```python
from build123d import *

# Parameters (mm, degrees)
BOSS_EXTRUDE1_DEPTH             = 52
BOSS_EXTRUDE2_DEPTH             = 22
BOSS_EXTRUDE3_DEPTH             = 12
F_1_0MM_CLEARANCE_DOWEL_HOLE1_D = 18
FILLET1_R                       = 15


with BuildPart() as part:
    # Sketch1 → Boss-Extrude1 (new body)
    with BuildSketch(Plane.XY):
        with BuildLine():
            Line((0, -34), (-108, -34))
            ThreePointArc((-108, -34), (-142, 0), (-108, 34))
            Line((-108, 34), (0, 34))
            ThreePointArc((0, 34), (34, 0), (0, -34))
        make_face()
        with BuildLine():
            Line((0, -15), (-108, -15))
            ThreePointArc((-108, -15), (-123, 0), (-108, 15))
            Line((-108, 15), (0, 15))
            ThreePointArc((0, 15), (15, 0), (0, -15))
        make_face(mode=Mode.SUBTRACT)
    extrude(amount=BOSS_EXTRUDE1_DEPTH)

    # Sketch2 → Boss-Extrude2 (add)
    with BuildSketch(Plane.XY):
        with BuildLine():
            Line((-126.998451924, 28.196787485), (0, 28.196787485))
            Line((0, 28.196787485), (31.319910556, 13.231145179))
            Line((31.319910556, 13.231145179), (31.319910556, 76))
            ThreePointArc((31.319910556, 76), (14.710725641, 103.650160006), (-17.500876911, 101.974143))
            Line((-17.500876911, 101.974143), (-126.998451924, 28.196787485))
        make_face()
    extrude(amount=BOSS_EXTRUDE2_DEPTH)

    # Sketch3 → Boss-Extrude3 (add)
    with BuildSketch(Plane.XY.offset(22)):
        with BuildLine():
            Line((-31.319910556, 76), (-31.319910556, 27.253285183))
            Line((-31.319910556, 27.253285183), (31.319910556, 13.231145179))
            Line((31.319910556, 13.231145179), (31.319910556, 76))
            ThreePointArc((31.319910556, 76), (0, 107.319910556), (-31.319910556, 76))
        make_face()
    extrude(amount=BOSS_EXTRUDE3_DEPTH)

    # Ø1.0mm Clearance Dowel Hole1 (through all)
    with Locations(Plane.XY.offset(34)):
        with Locations((0, 76)):
            Hole(F_1_0MM_CLEARANCE_DOWEL_HOLE1_D / 2)

    # Fillet1
    fillet1_edges = [part.edges().sort_by_distance(p)[0] for p in [
        (-31.319910556, 34, 28),
    ]]
    fillet(fillet1_edges, radius=FILLET1_R)


solid = part.part
```
The listing builds one solid part. Answer for the finished solid, in the listing's coordinates (mm). A direction names the side the tool comes from. Give positions to 0.01 mm unless a question says otherwise; leave off trailing zeros. Loops run counter-clockwise (first coordinate to the right, second up) from the corner with the lowest first, then second, coordinate; pieces in that order, holes last. Notation, with made-up numbers: M 64.5,30 L 76.5,30 A18 cw 76.5,65 Z; hole C -24.5,24.5 d2. An arc over 180 degrees is marked long. One line per item, written item: value.
Q1. For faces 1 (the face through (-35.6, 38.51, 27.92)), 2 (the face through (31.32, 44, 17)), 3 (the face through (15, 0, 26)), 4 (the face through (32.2, -10.92, 25.64)), determine the directions among +Z, -Z, +X, -X, +Y, -Y from which every point of the face is accessible in a straight line to the end or side of a thin tool.
Working result:
face 1: +Z, -X, +Y
face 2: +Z, -Z, +X, +Y
face 3: +Z, -Z
face 4: +Z, +X
Q2. A cutting plane is placed at A-A on y = 0. Determine the outline of the cut face in (x, z).
Working result:
outline: M -142,0 L -123,0 L -123,52 L -142,52 Z; M 15,0 L 34,0 L 34,52 L 15,52 Z
Q3. Find the intervals of material crossed by line 1 (Y direction, x = -6, z = 29); line 2 (X direction, y = -11, z = 32); line 3 (Z direction, x = -12, y = 74.5), in increasing order. Write a range as from..to.
Working result:
line 1: y = -34..-15, 15..69.29, 82.71..106.74
line 2: x = -140.17..-118.2, 10.2..32.17
line 3: z = 0..34
Q4. A cutting plane is placed at D-D on y = 87. Determine the outline of the cut face in (x, z).
Working result:
outline: M -39.72,0 L 29.32,0 L 29.32,34 L -29.32,34 L -29.32,22 L -39.72,22 Z
Q5. A cutting plane is placed at C-C on x = -104. Determine the outline of the cut face in (y, z), then the cut area to 3 significant figures.
Working result:
outline: M -34,0 L -15,0 L -15,52 L -34,52 Z; M 15,0 L 43.69,0 L 43.69,22 L 34,22 L 34,52 L 15,52 Z
area: 2,190 mm^2
Q6. Determine the mould class of faces 5 (the face through (-60, 54, 22)), 6 (the face through (1.951, 67.214, 16.762)), 7 (the face through (-141.99, -0.75, 25.64)) for opening direction Y: +Y half, -Y half, draft (parallel to the pull), parting line (faces both ways), or undercut.
Working result:
face 5: draft
face 6: undercut
face 7: parting line
Q7. Flat-ended cylindrical pins translate along their axes: P1, Ø3.5, axis at y = 69, z = 27.5, coming from the -X side; P2, Ø5, axis at x = -26.5, z = 44.5, coming from the +Y side; P3, Ø20.5, axis at x = 0, y = 76, coming from the +Z side. Find the tip coordinate at first contact, or state that the pin passes through.
Working result:
P1: stops at x = -31.32
P2: stops at y = 34
P3: stops at z = 34
Q8. A cutting plane is placed at B-B on z = 28. Determine the outline of the cut face in (x, y).
Working result:
outline: M -108,-34 L 0,-34 A34 ccw 31.32,13.23 L 31.32,76 A31.32 ccw -31.32,76 L -31.32,49 A15 cw -46.32,34 L -108,34 A34 ccw Z; hole M -108,-15 L 0,-15 A15 ccw 0,15 L -108,15 A15 ccw Z; hole C 0,76 d18
